```python
from build123d import *

# Parameters (mm, degrees)
SKETCH1_W           = 71
SKETCH1_H           = 121
SKETCH1_R           = 1.5
SKETCH1_R_2         = 11
BOSS_EXTRUDE1_DEPTH = 5
FILLET1_R           = 8


with BuildPart() as part:
    # Sketch1 → Boss-Extrude1 (new body)
    with BuildSketch(Plane(origin=(0, 0, 0), x_dir=(0, 0, -1), z_dir=(1, 0, 0))):
        with Locations((35.5, 60.5)):
            Rectangle(SKETCH1_W, SKETCH1_H)
        with Locations((6, 115)):
            Circle(SKETCH1_R, mode=Mode.SUBTRACT)
        with Locations((65, 115)):
            Circle(SKETCH1_R, mode=Mode.SUBTRACT)
        with Locations((35.5, 85.5)):
            Circle(SKETCH1_R_2, mode=Mode.SUBTRACT)
        with Locations((25.5, 95.5)):
            Circle(SKETCH1_R, mode=Mode.SUBTRACT)
        with Locations((45.5, 95.5)):
            Circle(SKETCH1_R, mode=Mode.SUBTRACT)
        with Locations((45.5, 75.5)):
            Circle(SKETCH1_R, mode=Mode.SUBTRACT)
        with Locations((25.5, 75.5)):
            Circle(SKETCH1_R, mode=Mode.SUBTRACT)
        with Locations((6, 56)):
            Circle(SKETCH1_R, mode=Mode.SUBTRACT)
        with Locations((65, 56)):
            Circle(SKETCH1_R, mode=Mode.SUBTRACT)
        with Locations((6, 6)):
            Circle(SKETCH1_R, mode=Mode.SUBTRACT)
        with Locations((65, 6)):
            Circle(SKETCH1_R, mode=Mode.SUBTRACT)
        with Locations((6, 46)):
            Circle(SKETCH1_R, mode=Mode.SUBTRACT)
        with Locations((65, 46)):
            Circle(SKETCH1_R, mode=Mode.SUBTRACT)
    extrude(amount=BOSS_EXTRUDE1_DEPTH)

    # Fillet1
    fillet1_edges = [part.edges().sort_by_distance(p)[0] for p in [
        (2.5, 121, 0),
        (2.5, 121, -71),
    ]]
    fillet(fillet1_edges, radius=FILLET1_R)


solid = part.part
```
Geometry check sheet. Reference: the model listing, model coordinates, mm. Give positions to 0.01 mm unless a question says otherwise; leave off trailing zeros. Order: outer loops, then holes, each group sorted by start corner. A loop starts at its lowest first (then second) coordinate and runs counter-clockwise, first axis right, second up. Notation, with made-up numbers: (-31.5, 80.25) - (23.5, 80.25) arc R16 cw to (23.5, 106.25) - close; hole circle Ø10 at (71.5, 79). An arc over 180 degrees is marked (long way). Answer in a Markdown table with one row per item. Add a question column.
Q1. Material ranges on probe 1 along Y at (x, z) = (3.1, -35.5); probe 2 along Y at (x, z) = (2.9, -64.5); probe 3 along Z at (x, y) = (1, 57), recorded low to high. Write a range as from..to.
Q2. Cross-section at B-B, the plane y = 46. Enter the section's corners in (x, z), then the cut area to 3 significant figures.
Q3. Cross-section at A-A, the plane z = -35.5. Enter the section's corners in (x, y), then the cut area to 3 significant figures.
Q4. Cross-section at D-D, the plane x = 3.55. Count the separate pieces of the cut face and the enclosed holes in it, then the cut area to 3 significant figures.
Q5. Cross-section at C-C, the plane y = 85.5. Enter the section's corners in (x, z), then the cut area to 3 significant figures.
Q6. Mould release check, pull along Y, two halves, no side actions. Record for faces 1 (the flat face through (2, 56, -71)), 2 (the cylindrical face through (2.465, 96.406, -34.068)), 3 (the cylindrical face through (2.535, 118.719, -68.594)): pulls with the +Y half, pulls with the -Y half, needs draft (parallel to the pull), parting line crosses it, or undercut.
Check values:
| question | item | result |
|---|---|---|
| 1 | probe 1 | y = 0..74.5, 96.5..121 |
| 1 | probe 2 | y = 0..4.59, 7.41..44.59, 47.41..54.59, 57.41..113.59, 116.41..120.86 |
| 1 | probe 3 | z = -71..-66.12, -63.88..-7.12, -4.88..0 |
| 2 | outline | (0, -71) - (5, -71) - (5, -66.5) - (0, -66.5) - close; (0, -63.5) - (5, -63.5) - (5, -7.5) - (0, -7.5) - close; (0, -4.5) - (5, -4.5) - (5, 0) - (0, 0) - close |
| 2 | area | 325 mm^2 |
| 3 | outline | (0, 0) - (5, 0) - (5, 74.5) - (0, 74.5) - close; (0, 96.5) - (5, 96.5) - (5, 121) - (0, 121) - close |
| 3 | area | 495 mm^2 |
| 4 | separate pieces | 1 |
| 4 | enclosed holes | 13 |
| 4 | area | 8,100 mm^2 |
| 5 | outline | (0, -71) - (5, -71) - (5, -46.5) - (0, -46.5) - close; (0, -24.5) - (5, -24.5) - (5, 0) - (0, 0) - close |
| 5 | area | 245 mm^2 |
| 6 | face 1 | needs draft |
| 6 | face 2 | undercut |
| 6 | face 3 | pulls with the +Y half |
